Can you work these out from the model? Positions are in its coordinate system, mm. Face numbers are marked on the shaded views. A direction names the side the tool comes from. Coordinates: 2 decimals unless noted, no trailing zeros. Loops run counter-clockwise (first coordinate to the right, second up) from the corner with the lowest first, then second, coordinate; pieces in that order, holes last. Notation, with made-up numbers: (-25, -12.5) -> (6, -12.5) arc R8 ccw to (6, -6.5) -> close; hole circle Ø3 at (79, 70.5). An arc over 180 degrees is marked (long way). Use one line per item in the form item = value. Start each with the question number.
(1) Thinking about a two-plate mould opening in Y: for the marked faces 3, 4, 5 and 6, which applies, released by +Y, released by -Y, zero draft, split by the parting line, or undercut?
(2) Imagine slicing it at C-C (x = 18). List the corners of the cut face in (y, z) for me.
(3) Imagine slicing it at D-D (y = 13). List the corners of the cut face in (x, z) for me, plus the area to 3 significant figures.
(4) Imagine slicing it at B-B (z = 3.75). List the corners of the cut face in (x, y) for me, plus the area to 3 significant figures.
(5) I'm going to push a flat-ended pin straight in: pin 1 (15.5 mm diameter, centred on x = 26.58, y = -8.16, fed in from +Z). Where does the tip first touch, or does it pass through?
(6) Imagine slicing it at A-A (y = -3). List the corners of the cut face in (x, z) for me, plus the area to 3 significant figures.
(7) On a 3-axis mill with a long thin cutter (end or side, diameter ignored), from which of +Z, -Z, +X, -X, +Y, -Y can I reach the whole of each face in a straight line? I mean the marked faces 1 and 2. Say none if no direction works.
(8) I need wall thicknesses on line 1 (Y direction, x = 27, z = 6.5); line 2 (X direction, y = 5.5, z = 4); line 3 (Z direction, x = -10, y = -6). Which ranges of each line are inside material? Lowest first, please. Write a range as [from, to].
```python
from build123d import *

# Parameters (mm, degrees)
F0_W         = 76.2
F0_H         = 37.856084797
F1_DEPTH     = 7.62
F2_R         = 1.27
F3_T1_DEPTH  = 20.32
F3_T4_ANGLE  = 90
F3_T6_ANGLE  = 90
F3_T8_ANGLE  = 90
F3_T10_ANGLE = 90
F5_DEPTH     = 25.4
F6_R         = 5.9846476777
F7_DEPTH     = 25.4
F10_DEPTH    = 12.7


# Not quite as in the source:
# - a fillet or chamfer that OpenCascade refuses, or shapes differently, is made with other operations: its cross-section is extruded or revolved along the edge and cut away or added


with BuildPart() as f1:
    # F0 (on Top) → F1 (new body)
    with BuildSketch(Plane.XY):
        Rectangle(F0_W, F0_H)
    extrude(amount=F1_DEPTH)

    # F2
    f2_edges = [f1.edges().sort_by_distance(p)[0] for p in [
        (-38.1, 0, 7.62),
        (0, 18.928042, 7.62),
        (38.1, 0, 7.62),
        (0, -18.928042, 7.62),
    ]]
    fillet(f2_edges, radius=F2_R)

    # F3: fillet of radius 5.08 on 4 edges, made by hand

    # F3_s2 → F3_t1 (cut)
    with BuildSketch(Plane.XY.offset(-12.7)):
        with BuildLine():
            ThreePointArc((-33.02, -18.9280423985), (-36.6121024484, -17.4401448469), (-38.1, -13.8480423985))
            Line((-38.1, -13.8480423985), (-38.1, -18.9280423985))
            Line((-38.1, -18.9280423985), (-33.02, -18.9280423985))
        make_face()
        with BuildLine():
            ThreePointArc((-33.02, 18.9280423985), (-36.6121024484, 17.4401448469), (-38.1, 13.8480423985))
            Line((-38.1, 13.8480423985), (-38.1, 18.9280423985))
            Line((-38.1, 18.9280423985), (-33.02, 18.9280423985))
        make_face()
        with BuildLine():
            ThreePointArc((38.1, 13.8480423985), (36.6121024484, 17.4401448469), (33.02, 18.9280423985))
            Line((33.02, 18.9280423985), (38.1, 18.9280423985))
            Line((38.1, 18.9280423985), (38.1, 13.8480423985))
        make_face()
        with BuildLine():
            ThreePointArc((38.1, -13.8480423985), (36.6121024484, -17.4401448469), (33.02, -18.9280423985))
            Line((33.02, -18.9280423985), (38.1, -18.9280423985))
            Line((38.1, -18.9280423985), (38.1, -13.8480423985))
        make_face()
    extrude(amount=F3_T1_DEPTH, mode=Mode.SUBTRACT)

    # F3_s3 → F3_t4 (revolve, cut)
    with BuildSketch(Plane.YZ.offset(33.02)):
        with BuildLine():
            ThreePointArc((-17.6580423985, 7.62), (-18.5560680106, 7.2480256121), (-18.9280423985, 6.35))
            Line((-18.9280423985, 6.35), (-18.9280423985, 7.62))
            Line((-18.9280423985, 7.62), (-17.6580423985, 7.62))
        make_face()
    revolve(axis=Axis((33.02, -13.8480423985, 7.62), (0, 0, 1)), revolution_arc=F3_T4_ANGLE, mode=Mode.SUBTRACT)

    # F3_s5 → F3_t6 (revolve, cut)
    with BuildSketch(Plane.XZ.offset(-13.8480423985)):
        with BuildLine():
            ThreePointArc((36.83, 7.62), (37.7280256121, 7.2480256121), (38.1, 6.35))
            Line((38.1, 6.35), (38.1, 7.62))
            Line((38.1, 7.62), (36.83, 7.62))
        make_face()
    revolve(axis=Axis((33.02, 13.8480423985, 7.62), (0, 0, 1)), revolution_arc=F3_T6_ANGLE, mode=Mode.SUBTRACT)

    # F3_s7 → F3_t8 (revolve, cut)
    with BuildSketch(Plane.YZ.offset(-33.02)):
        with BuildLine():
            ThreePointArc((17.6580423985, 7.62), (18.5560680106, 7.2480256121), (18.9280423985, 6.35))
            Line((18.9280423985, 6.35), (18.9280423985, 7.62))
            Line((18.9280423985, 7.62), (17.6580423985, 7.62))
        make_face()
    revolve(axis=Axis((-33.02, 13.8480423985, 7.62), (0, 0, 1)), revolution_arc=F3_T8_ANGLE, mode=Mode.SUBTRACT)

    # F3_s9 → F3_t10 (revolve, cut)
    with BuildSketch(Plane.XZ.offset(13.8480423985)):
        with BuildLine():
            ThreePointArc((-36.83, 7.62), (-37.7280256121, 7.2480256121), (-38.1, 6.35))
            Line((-38.1, 6.35), (-38.1, 7.62))
            Line((-38.1, 7.62), (-36.83, 7.62))
        make_face()
    revolve(axis=Axis((-33.02, -13.8480423985, 7.62), (0, 0, 1)), revolution_arc=F3_T10_ANGLE, mode=Mode.SUBTRACT)

    # F4 (on face) → F5 (cut)
    with BuildSketch(Plane.XY.offset(7.62)):
        with BuildLine():
            Line((-29.6291131526, 8.6681647226), (-29.6291131526, 0))
            Line((-29.6291131526, 0), (-29.6291131526, -8.6681647226))
            ThreePointArc((-29.6291131526, -8.6681647226), (-26.7311763018, -11.5661015734), (-23.8332394511, -8.6681647226))
            Line((-23.8332394511, -8.6681647226), (-23.8332394511, 0))
            Line((-23.8332394511, 0), (-23.8332394511, 8.6681647226))
            ThreePointArc((-23.8332394511, 8.6681647226), (-26.7311763018, 11.5661015734), (-29.6291131526, 8.6681647226))
        make_face()
    extrude(amount=-F5_DEPTH, mode=Mode.SUBTRACT)

    # F6 (on face) → F7 (cut)
    with BuildSketch(Plane.XY.offset(7.62)):
        with Locations((26.5783518553, -8.1568043679)):
            Circle(F6_R)
    extrude(amount=-F7_DEPTH, mode=Mode.SUBTRACT)

    # F9 (on face) → F10 (join, symmetric)
    with BuildSketch(Plane(origin=(-7.5825373642, -7.5825373642, 0), x_dir=(-0.7071067812, 0.7071067812, 0), z_dir=(0.7071067812, 0.7071067812, 0))):
        Polygon((4.9822961397, 7.62), (10.2810509175, 20.9576525145), (8.66903996, 21.5980688662), (3.1158619095, 7.62), align=None)
    extrude(amount=F10_DEPTH, both=True)


solid = f1.part
```
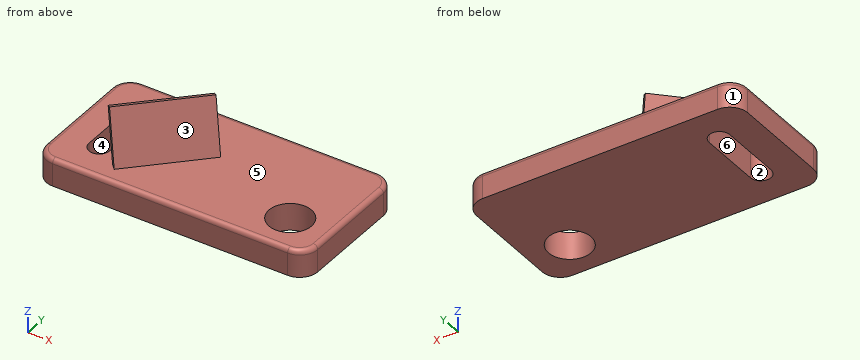
Worked out:
q1.face_3 = released by -Y
q1.face_4 = undercut
q1.face_5 = zero draft
q1.face_6 = undercut
q2.outline = (-18.93, 0) -> (18.93, 0) -> (18.93, 6.35) arc R1.27 ccw to (17.66, 7.62) -> (-17.66, 7.62) arc R1.27 ccw to (-18.93, 6.35) -> close
q3.outline = (-38.1, 0) -> (38.1, 0) -> (38.1, 6.35) arc R1.27 ccw to (36.83, 7.62) -> (-36.83, 7.62) arc R1.27 ccw to (-38.1, 6.35) -> close
q3.area = 580 mm2
q4.outline = (-38.1, -13.85) arc R5.08 ccw to (-33.02, -18.93) -> (33.02, -18.93) arc R5.08 ccw to (38.1, -13.85) -> (38.1, 13.85) arc R5.08 ccw to (33.02, 18.93) -> (-33.02, 18.93) arc R5.08 ccw to (-38.1, 13.85) -> close; hole (-29.63, -8.67) arc R2.9 ccw to (-23.83, -8.67) -> (-23.83, 8.67) arc R2.9 ccw to (-29.63, 8.67) -> close; hole circle Ø11.97 at (26.58, -8.16)
q4.area = 2,620 mm2
q5.pin_1 = 7.62
q6.outline = (-38.1, 0) -> (-29.63, 0) -> (-29.63, 7.62) -> (-36.83, 7.62) arc R1.27 ccw to (-38.1, 6.35) -> close; (-23.83, 0) -> (23.54, 0) -> (23.54, 7.62) -> (-7.41, 7.62) -> (-15.26, 21.6) -> (-17.54, 20.96) -> (-10.05, 7.62) -> (-23.83, 7.62) -> close; (29.62, 0) -> (38.1, 0) -> (38.1, 6.35) arc R1.27 ccw to (36.83, 7.62) -> (29.62, 7.62) -> close
q6.area = 526 mm2
q7.face_1 = +Z, -Z, -X, +Y
q7.face_2 = +Z, -Z
q8.line_1 = [-18.92, -14.13], [-2.19, 18.92]
q8.line_2 = [-38.1, -29.63], [-23.83, 38.1]
q8.line_3 = [0, 7.62]
